Here's how the part is built. I have some questions about the finished solid (model axes, mm). Face numbers are marked on the shaded views. A direction names the side the tool comes from. Give positions to 0.01 mm unless a question says otherwise; leave off trailing zeros. Loops run counter-clockwise (first coordinate to the right, second up) from the corner with the lowest first, then second, coordinate; pieces in that order, holes last. Notation, with made-up numbers: M -3.5,17.5 L 36.5,17.5 A28 ccw 36.5,50.5 Z; hole C 28.25,30.5 d9. An arc over 180 degrees is marked long. Write item = value, one per line. Start each with the question number.
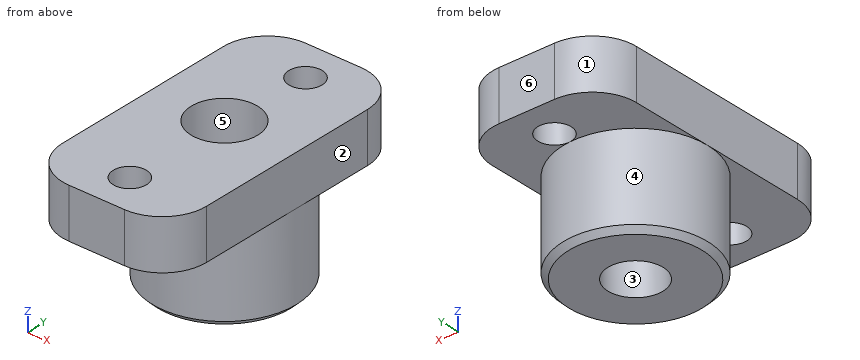
Autodesk Inventor part; units mm, degrees
ref_plane "YZ Plane" through (0, 0, 0) normal (1, 0, 0) x (0, 1, 0)
ref_plane "XZ Plane" through (0, 0, 0) normal (0, 1, 0) x (-1, 0, 0)
ref_plane "XY Plane" through (0, 0, 0) normal (0, 0, 1) x (1, 0, 0)
sketch "Skizze1" plane through (0, 0, 0) normal (0, 0, 1) x (1, 0, 0)
  line L0 (-6.5, 13.5) -> (6.5, 13.5)
  line L1 (6.5, 13.5) -> (6.5, -13.5)
  line L2 (6.5, -13.5) -> (-6.5, -13.5)
  line L3 (-6.5, -13.5) -> (-6.5, 13.5)
  line L4 (-6.5, 13.5) -> (6.5, -13.5) construction
  line L5 (6.5, 13.5) -> (-6.5, -13.5) construction
  line L6 (0, 0) -> (0.502324, 7.984214) construction
  line L7 (0, 0) -> (0, -13.5) construction
  circle A0 centre (0, -10) radius 1.5
  circle A1 centre (0.502324, 7.984214) radius 1.5
  line L8 (-6.5, 11.5) -> (6.5, 11.5)
  circle A2 centre (0, 0) radius 6.5
  circle A3 centre (0, 0) radius 2.475
  circle A4 centre (0, 0) radius 1.35
  circle A5 centre (0, 0) radius 3
  dimension "d13" = 3
  dimension "d14" = 3
  dimension "d15" = 3.5
  dimension "d16" = 10
  dimension "d17" = 8
  dimension "d18" = 3.6
  dimension "d23" = 4.95
  dimension "d26" = 2.7
  dimension "d29" = 6
  dimension "d37" = 13
  dimension "d39" = 25
extrude "Extrusion1" add sketch "Skizze1" along normal blind 4.5 contours L8 L1 A2 L3 | A2 L1 L2 L3 | A2 | A3 | A4 | A5
extrude "Extrusion2" add sketch "Skizze1" against normal blind 8.2 contours A2 | A5
extrude "Extrusion3" cut sketch "Skizze1" along normal through all contours A4
extrude "Extrusion4" cut sketch "Skizze1" against normal blind 7 from surface at 4.5 contours A3 | A4 | A5
chamfer "Fase1" distance 0.5 angle 45 1 edges at (-6.5, 0, -8.2)
fillet "Rundung1" radius 4 4 edges at (6.5, 11.5, 2.25) (-6.5, 11.5, 2.25) (6.5, -13.5, 2.25) (-6.5, -13.5, 2.25)
extrude "Extrusion6" add sketch "Skizze1" against normal blind 4.95 contours A3 | A5
extrude "Extrusion7" cut sketch "Skizze1" against normal blind 1 contours A3 | A5
equation "\"d14\" = d13"
properties part number "daVinci_Tool_Clutch"
Q1. If we section it at C-C, the plane y = -10: List the corners of the cut face in (x, z) for me, then the cut area to 3 significant figures.
Q2. Will these pins go through, and if not, where does the flat tip stop? pin 1 (2.5 mm diameter, centred on x = 0, y = 0, fed in from -Z); pin 2 (2.5 mm diameter, centred on x = 1, y = -0.5, fed in from -Z); pin 3 (1.5 mm diameter, centred on y = -1.5, z = -3, fed in from -X); pin 4 (2 mm diameter, centred on y = -6.5, z = -5, fed in from -X).
Q3. On a 3-axis mill with a long thin cutter (end or side, diameter ignored), from which of +Z, -Z, +X, -X, +Y, -Y can I reach the whole of each face in a straight line? I mean the marked faces 4, 5 and 6. Say none if no direction works.
Q4. We'd pull the mould along X, two halves only. Please class the marked faces 1, 2 and 3: pulls with the +X half, pulls with the -X half, needs draft (parallel to the pull), parting line crosses it, or undercut.
Q5. If we section it at A-A, the plane x = 0: State how many separate pieces and enclosed holes the cut face has, then the cut area to 3 significant figures.
Q6. If we section it at B-B, the plane z = -0.5: List the corners of the cut face in (x, y) for me, then the cut area to 3 significant figures.
Q7. If we section it at D-D, the plane y = 10.25: List the corners of the cut face in (x, z) for me.
Q8. If I drill on line 1 along Y through (x, z) = (0, -6.45) (3 decimals); line 2 along Z through (x, y) = (3, -7); line 3 along Y through (x, z) = (0, -2.95), over which ranges is the centre line in solid material (lowest first)?
Resolved:
q1.outline = M -6.47,0 L -1.5,0 L -1.5,4.5 L -6.47,4.5 Z; M 1.5,0 L 6.47,0 L 6.47,4.5 L 1.5,4.5 Z
q1.area = 44.7 mm²
q2.pin_1 = through
q2.pin_2 = -4.95
q2.pin_3 = -6.46
q2.pin_4 = -3.46
q3.face_4 = -Z
q3.face_5 = +Z
q3.face_6 = +Z, -Z, +X, -X, +Y
q4.face_1 = pulls with the -X half
q4.face_2 = pulls with the +X half
q4.face_3 = undercut
q5.separate_pieces = 4
q5.enclosed_holes = 0
q5.area = 133 mm²
q6.outline = C 0,0 d13; hole C 0,0 d6
q6.area = 104 mm²
q7.outline = M -5.4,0 L 5.4,0 L 5.4,4.5 L -5.4,4.5 Z
q8.line_1 = -6.5 to -2.475, 2.475 to 6.5
q8.line_2 = 0 to 4.5
q8.line_3 = -6.5 to -1.35, 1.35 to 6.5
